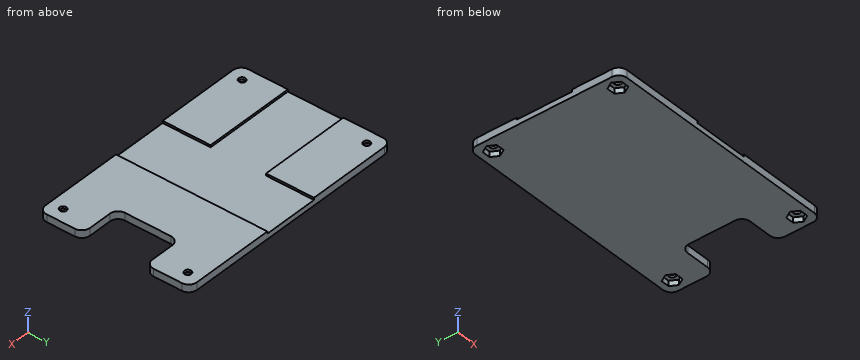
from build123d import *

# Parameters (mm, degrees)
F1_DEPTH = 2.667
F2_R     = 1.2192
F3_DEPTH = 2.668
F5_DEPTH = 1.8415
F7_DEPTH = 0.762
F9_DEPTH = 2.668
F10_R    = 2.921


with BuildPart() as f1:
    # F0 (on Top) → F1 (new body)
    with BuildSketch(Plane.XY):
        with BuildLine():
            Line((39.85895, 27.0002), (-39.85895, 27.0002))
            ThreePointArc((-39.85895, 27.0002), (-41.9244089078, 26.1446589078), (-42.77995, 24.0792))
            Line((-42.77995, 24.0792), (-42.77995, -24.0792))
            ThreePointArc((-42.77995, -24.0792), (-41.9244089078, -26.1446589078), (-39.85895, -27.0002))
            Line((-39.85895, -27.0002), (39.85895, -27.0002))
            ThreePointArc((39.85895, -27.0002), (41.9244089078, -26.1446589078), (42.77995, -24.0792))
            Line((42.77995, -24.0792), (42.77995, 24.0792))
            ThreePointArc((42.77995, 24.0792), (41.9244089078, 26.1446589078), (39.85895, 27.0002))
        make_face()
    extrude(amount=F1_DEPTH)

    # F2 (on face) → F3 (cut, through all)
    with BuildSketch(Plane(origin=(0, 0, 0), x_dir=(1, 0, 0), z_dir=(0, 0, -1))):
        with Locations((-38.01745, 22.2377)):
            Circle(F2_R)
        with Locations((-38.01745, -22.2377)):
            Circle(F2_R)
        with Locations((38.01745, -22.2377)):
            Circle(F2_R)
        with Locations((38.01745, 22.2377)):
            Circle(F2_R)
    extrude(amount=-F3_DEPTH, mode=Mode.SUBTRACT)

    # F4 (on face) → F5 (cut)
    with BuildSketch(Plane(origin=(0, 0, 0), x_dir=(1, 0, 0), z_dir=(0, 0, -1))):
        Polygon((-36.5693111873, 19.72945), (-35.1211723746, 22.2377), (-36.5693111873, 24.74595), (-39.4655888127, 24.74595), (-40.9137276254, 22.2377), (-39.4655888127, 19.72945), align=None)
        Polygon((-35.1211723746, -22.2377), (-36.5693111873, -19.72945), (-39.4655888127, -19.72945), (-40.9137276254, -22.2377), (-39.4655888127, -24.74595), (-36.5693111873, -24.74595), align=None)
        Polygon((35.1211723746, 22.2377), (36.5693111873, 19.72945), (39.4655888127, 19.72945), (40.9137276254, 22.2377), (39.4655888127, 24.74595), (36.5693111873, 24.74595), align=None)
        Polygon((36.5693111873, -19.72945), (35.1211723746, -22.2377), (36.5693111873, -24.74595), (39.4655888127, -24.74595), (40.9137276254, -22.2377), (39.4655888127, -19.72945), align=None)
    extrude(amount=-F5_DEPTH, mode=Mode.SUBTRACT)

    # F6 (on face) → F7 (cut)
    with BuildSketch(Plane.XY.offset(2.667)):
        Polygon((9.906, 27.0002), (-9.906, 27.0002), (-9.906, 9.906), (-42.77995, 9.906), (-42.77995, -9.906), (-9.906, -9.906), (-9.906, -27.0002), (9.906, -27.0002), align=None)
    extrude(amount=-F7_DEPTH, mode=Mode.SUBTRACT)

    # F8 (on face) → F9 (cut, through all)
    with BuildSketch(Plane.XY.offset(2.667)):
        with BuildLine():
            Line((57.06745, 11.1125), (31.41345, 11.1125))
            ThreePointArc((31.41345, 11.1125), (29.3479910922, 10.2569589078), (28.49245, 8.1915))
            Line((28.49245, 8.1915), (28.49245, -8.1915))
            ThreePointArc((28.49245, -8.1915), (29.3479910922, -10.2569589078), (31.41345, -11.1125))
            Line((31.41345, -11.1125), (57.06745, -11.1125))
            Line((57.06745, -11.1125), (57.06745, 11.1125))
        make_face()
    extrude(amount=-F9_DEPTH, mode=Mode.SUBTRACT)

    # F10
    f10_edges = [f1.edges().sort_by_distance(p)[0] for p in [
        (42.77995, 11.1125, 1.3335),
        (42.77995, -11.1125, 1.3335),
    ]]
    fillet(f10_edges, radius=F10_R)


solid = f1.part
Check sheet for the modelled part. Datum: model origin and axes. Units: mm. Give positions to 0.01 mm unless a question says otherwise; leave off trailing zeros. Loops run counter-clockwise (first coordinate to the right, second up) from the corner with the lowest first, then second, coordinate; pieces in that order, holes last. Notation, with made-up numbers: M 78,-9.5 L 93,-9.5 A27 cw 93,17.5 Z; hole C -39.5,75 d8. An arc over 180 degrees is marked long. Use a Markdown table: item, result. Add a question column.
Q1. Sectioned sample at B-B, the plane y = 18.5. Record the cut outline in (x, z) (3 decimals).
Q2. Sectioned sample at A-A, the plane x = 34. Record the cut outline in (y, z).
Q3. Sectioned sample at D-D, the plane x = 2.5. Record the cut outline in (y, z) (3 decimals), then the cut area to 3 significant figures.
Q4. Sectioned sample at C-C, the plane z = 0.45. Give the number of separate pieces and of enclosed holes in the cut face, then the cut area to 3 significant figures.
Q5. Go/stop test with flat-tipped pins: pin 1 (1.5 mm diameter, centred on y = -4, z = 1, fed in from +X); pin 2 (3 mm diameter, centred on x = -38.02, y = 22.24, fed in from -Z); pin 3 (1.5 mm diameter, centred on x = -38.02, y = -22.24, fed in from +Z). Record where each tip stops, or that it passes through.
Q6. Scan lines: line 1 along Y through (x, z) = (36.5, 0.8); line 2 along X through (y, z) = (23.5, 1.5); line 3 along X through (y, z) = (0, 1.45). Record each from-to range of solid material in increasing order. Write a range as [from, to].
Verdict:
| question | item | result |
|---|---|---|
| 1 | outline | M -42.78,0 L 42.78,0 L 42.78,2.667 L 9.906,2.667 L 9.906,1.905 L -9.906,1.905 L -9.906,2.667 L -42.78,2.667 Z |
| 2 | outline | M -27,0 L -11.11,0 L -11.11,2.67 L -27,2.67 Z; M 11.11,0 L 27,0 L 27,2.67 L 11.11,2.67 Z |
| 3 | outline | M -27,0 L 27,0 L 27,1.905 L -27,1.905 Z |
| 3 | area | 103 mm^2 |
| 4 | separate pieces | 1 |
| 4 | enclosed holes | 4 |
| 4 | area | 4,210 mm^2 |
| 5 | pin 1 | x = 28.49 |
| 5 | pin 2 | z = 1.84 |
| 5 | pin 3 | through |
| 6 | line 1 | [-27, -24.63], [-19.85, -11.11], [11.11, 19.85], [24.63, 27] |
| 6 | line 2 | [-42.78, -40.18], [-35.85, 35.85], [40.18, 42.78] |
| 6 | line 3 | [-42.78, 28.49] |
